from build123d import *

# Parameters (mm, degrees)
SKETCH1_R           = 34.925
EXTRUDE1_DEPTH      = 30.1498
EXTRUDE1_DEPTH_BACK = 119.0752
CUT_EXTRUDE1_REACH  = 121.075
SKETCH2_R           = 34.925
SKETCH2_R_2         = 31.496
CUT_EXTRUDE3_START  = -30.1498
SKETCH4_R           = 41.275
CUT_EXTRUDE3_DEPTH  = 30.1498
SKETCH18_R          = 9.525
CUT_EXTRUDE4_DEPTH  = 0.254
SKETCH19_R          = 9.525
CUT_EXTRUDE5_DEPTH  = 0.254
CHAMFER1_SIZE       = 0.762
SKETCH15_R          = 6.9469
EXTRUDE2_DEPTH      = 1.27
CIRPATTERN1_COUNT   = 4


with BuildPart() as part:
    # Sketch1 → Extrude1 (new body, two sides)
    with BuildSketch(Plane(origin=(0, 0, 0), x_dir=(0, 0, -1), z_dir=(1, 0, 0))) as extrude1_sk:
        Circle(SKETCH1_R)
    extrude(amount=EXTRUDE1_DEPTH)
    extrude(extrude1_sk.sketch, amount=-EXTRUDE1_DEPTH_BACK)

    # Sketch2 → Cut-Extrude1 (cut, up to next)
    with BuildSketch(Plane(origin=(0, 0, 0), x_dir=(0, 0, -1), z_dir=(1, 0, 0)), mode=Mode.PRIVATE) as cut_extrude1_sk1:
        Circle(SKETCH2_R)
        with Locations((0, -2.54)):
            Circle(SKETCH2_R_2, mode=Mode.SUBTRACT)
    cut_extrude1_tool1 = extrude(cut_extrude1_sk1.sketch, amount=-CUT_EXTRUDE1_REACH, mode=Mode.PRIVATE) & part.part
    add(cut_extrude1_tool1.solids().sort_by_distance((0, 0, 33.937172))[0], mode=Mode.SUBTRACT)

    # Sketch4 → Cut-Extrude3 (cut)
    with BuildSketch(Plane.ZY.offset(CUT_EXTRUDE3_START)):
        Circle(SKETCH4_R)
        with BuildLine():
            Line((31.623, -14.823680245), (31.623, 20.938179637))
            Line((31.623, 20.938179637), (0, 39.195727199))
            Line((0, 39.195727199), (-31.623, 20.938179637))
            Line((-31.623, 20.938179637), (-31.623, -14.823680245))
            ThreePointArc((-31.623, -14.823680245), (0, -34.925), (31.623, -14.823680245))
        make_face(mode=Mode.SUBTRACT)
    extrude(amount=CUT_EXTRUDE3_DEPTH, mode=Mode.SUBTRACT)

    # Sketch6 → Cut-Revolve2 (revolve, cut)
    with BuildSketch(Plane.XY, mode=Mode.PRIVATE) as cut_revolve2_sk:
        Polygon((0.307141936, 69.85), (30.1498, 18.161), (30.1498, 69.85), align=None)
    revolve(cut_revolve2_sk.sketch.rotate(Axis((-1.184990967, -2.54, 0), (1, 0, 0)), 270), axis=Axis((-1.184990967, -2.54, 0), (1, 0, 0)), mode=Mode.SUBTRACT)  # turned: the seam where the file's is

    # S2D0002 → Cut-Revolve3 (revolve, cut)
    with BuildSketch(Plane(origin=(9.9568, 29.176824947, 16.845247737), x_dir=(0, 0.5, -0.866025404), z_dir=(1, 0, 0))):
        Polygon((0, 0), (6.1849, 0), (5.642306865, -2.5527), (4.9784, -3.216606865), (4.9784, -13.462), (0, -13.462), align=None)
    revolve(axis=Axis((9.9568, 16.935469262, 9.777697737), (0, 0.866025404, 0.5)), mode=Mode.SUBTRACT)

    # Sketch8 → Cut-Revolve4 (revolve, cut)
    with BuildSketch(Plane(origin=(9.9568, 29.176824947, -16.845247737), x_dir=(0, -0.5, -0.866025404), z_dir=(1, 0, 0))):
        Polygon((0, 0), (6.1849, 0), (5.642306865, -2.5527), (4.9784, -3.216606865), (4.9784, -13.462), (0, -13.462), align=None)
    revolve(axis=Axis((9.9568, 16.935469262, -9.777697737), (0, 0.866025404, -0.5)), mode=Mode.SUBTRACT)

    # Sketch18 → Cut-Extrude4 (cut)
    with BuildSketch(Plane(origin=(0, 29.396795399, 16.972247737), x_dir=(1, 0, 0), z_dir=(0, 0.866025404, 0.5))):
        with Locations((9.9568, 0)):
            Circle(SKETCH18_R)
    extrude(amount=-CUT_EXTRUDE4_DEPTH, mode=Mode.SUBTRACT)

    # Sketch19 → Cut-Extrude5 (cut)
    with BuildSketch(Plane(origin=(0, 29.396795399, -16.972247737), x_dir=(1, 0, 0), z_dir=(0, 0.866025404, -0.5))):
        with Locations((9.9568, 0)):
            Circle(SKETCH19_R)
    extrude(amount=-CUT_EXTRUDE5_DEPTH, mode=Mode.SUBTRACT)

    # Sketch10 → Cut-Revolve6 (revolve, cut)
    with BuildSketch(Plane.XY, mode=Mode.PRIVATE) as cut_revolve6_sk:
        Polygon((0, 28.956), (0, 28.067), (-3.81, 28.067), (-4.699, 28.956), align=None)
    revolve(cut_revolve6_sk.sketch.rotate(Axis((-4.93395, -2.54, 0), (1, 0, 0)), 90), axis=Axis((-4.93395, -2.54, 0), (1, 0, 0)), mode=Mode.SUBTRACT)  # turned: the seam where the file's is

    # Sketch12 → Cut-Revolve8 (revolve, cut)
    with BuildSketch(Plane.XY, mode=Mode.PRIVATE) as cut_revolve8_sk:
        Polygon((-119.0752, 28.956), (-119.0752, 28.067), (-116.5352, 28.067), (-115.6462, 28.956), align=None)
    revolve(cut_revolve8_sk.sketch.rotate(Axis((-119.24665, -2.54, 0), (1, 0, 0)), 90), axis=Axis((-119.24665, -2.54, 0), (1, 0, 0)), mode=Mode.SUBTRACT)  # turned: the seam where the file's is

    # Chamfer1
    chamfer1_edges = [part.edges().sort_by_distance(p)[0] for p in [
        (-119.0752, -2.54, -30.607),
    ]]
    chamfer(chamfer1_edges, length=CHAMFER1_SIZE)

    # Sketch13 → Revolve1 (revolve)
    with BuildSketch(Plane(origin=(0, 0, 0), x_dir=(0, -1, 0), z_dir=(0, 0, 1)), mode=Mode.PRIVATE) as revolve1_sk:
        with BuildLine():
            Line((2.54, 30.1498), (2.54, 82.7786))
            Line((2.54, 82.7786), (17.399, 82.7786))
            ThreePointArc((17.399, 82.7786), (18.11742049, 82.48102049), (18.415, 81.7626))
            Line((18.415, 81.7626), (18.415, 30.1498))
            Line((18.415, 30.1498), (2.54, 30.1498))
        make_face()
    revolve(revolve1_sk.sketch.rotate(Axis((27.51836, -2.54, 0), (1, 0, 0)), 270), axis=Axis((27.51836, -2.54, 0), (1, 0, 0)))  # turned: the seam where the file's is

    # S2D0001 → Cut-Revolve9 (revolve, cut)
    with BuildSketch(Plane(origin=(82.7786, -9.8806, 0), x_dir=(0, -1, 0), z_dir=(0, 0, 1)), mode=Mode.PRIVATE) as cut_revolve9_sk:
        Polygon((0, 0), (0, -25.4), (-7.3406, -29.81067746), (-7.3406, 0), align=None)
    revolve(cut_revolve9_sk.sketch.rotate(Axis((51.477388667, -2.54, 0), (1, 0, 0)), 270), axis=Axis((51.477388667, -2.54, 0), (1, 0, 0)), mode=Mode.SUBTRACT)  # turned: the seam where the file's is

    # Sketch15 → Extrude2 (add)
    with BuildSketch(Plane(origin=(30.1498, 29.176824947, -16.845247737), x_dir=(0, -0.5, -0.866025404), z_dir=(0, -0.866025404, 0.5))):
        with Locations((0, -20.193)):
            Circle(SKETCH15_R)
    extrude(amount=-EXTRUDE2_DEPTH)

    # Sketch16 → Cut-Revolve10 (revolve, cut)
    with BuildSketch(Plane(origin=(78.8162, 8.685320151, -11.225320151), x_dir=(-1, 0, 0), z_dir=(0, -0.707106781, -0.707106781)), mode=Mode.PRIVATE) as cut_revolve10_sk:
        Polygon((0, 0), (2.413, 0), (0, -2.413), align=None)
    cut_revolve10 = revolve(cut_revolve10_sk.sketch.rotate(Axis((78.8162, 6.893759055, -9.433759055), (0, 0.707106781, -0.707106781)), 90), axis=Axis((78.8162, 6.893759055, -9.433759055), (0, 0.707106781, -0.707106781)), mode=Mode.SUBTRACT)  # turned: the seam where the file's is

    # CirPattern1: Cut-Revolve10 ×4 about axis
    cirpattern1_axis = Axis((27.51836, -2.54, 0), (-1, 0, 0))
    for i in range(1, CIRPATTERN1_COUNT):
        add(cut_revolve10.rotate(cirpattern1_axis, i * 360 / CIRPATTERN1_COUNT), mode=Mode.SUBTRACT)


solid = part.part
Input: part model. Units: mm. Frame: model coordinates. A direction names the side the tool comes from. Give positions to 0.01 mm unless a question says otherwise; leave off trailing zeros. Loops run counter-clockwise (first coordinate to the right, second up) from the corner with the lowest first, then second, coordinate; pieces in that order, holes last. Notation, with made-up numbers: (5, 89) -> (51, 89) arc R21 ccw to (51, 97) -> close; hole circle Ø2 at (31, 51.25). An arc over 180 degrees is marked (long way). Answer as a JSON object with one key per item and string values. Group by question number.
Item 1: Pin query (flat end, axial travel): P1, Ø1.5, axis at x = -53.5, y = 14.5, coming from the +Z side; P2, Ø17, axis at y = -2.54, z = 0, coming from the +X side; P3, Ø1.5, axis at x = -23.5, z = 10.5, coming from the -Y side; P4, Ø10, axis at x = 35.5, z = 8, coming from the +Y side. Return the tip coordinate at first contact, or that it passes through.
Item 2: Pull-direction query (Z, two-part tool) for faces 1 (the flat face through (14.06, 32.18, -11.64)), 2 (the flat face through (12, 0, -31.623)), 3 (the cylindrical face through (10.79, 20.48, 28.29)); classes: released by +Z, released by -Z, zero draft, split by the parting line, or undercut.
Item 3: Reachability of faces 4 (the cylindrical face through (69.901, 1.927, -5.825)), 5 (the flat face through (20.2, 29.34, 17.07)), 6 (the flat face through (9.887, 17.484, 10.175)), 7 (the flat face through (0.298, 29.112, -17.466)) from +Z, -Z, +X, -X, +Y, -Y: full face, straight path, thin tool, end or side. Return the list, or none.
Item 4: Line query: probe 1 along Y at (x, z) = (69, 0) (3 decimals); probe 2 along Z at (x, y) = (67, -2); probe 3 along X at (y, z) = (-18, -5.5). Output: solid intervals per line, ascending.
Item 5: Cut plane A-A, the plane x = -63. Return the cut outline in (y, z).
Checks:
{
 "1": {"P1": "stops at z = 26.96", "P2": "stops at x = 82.78", "P3": "stops at y = -32.49", "P4": "stops at y = 13.05"},
 "2": {"face 1": "undercut", "face 2": "released by -Z", "face 3": "released by +Z"},
 "3": {"face 4": "+X", "face 5": "+Z, +X, -X, +Y", "face 6": "none", "face 7": "-Z, -X, +Y"},
 "4": {"probe 1": "y = -18.415 to -9.881, 4.801 to 13.335", "probe 2": "z = -15.87 to -7.32, 7.32 to 15.87", "probe 3": "x = -119.08 to 30.15"},
 "5": {"outline": "circle Ø62.99 at (-2.54, 0)"}
}
